from build123d import *

# Parameters (mm, degrees)
PAD_DEPTH       = 10
SKETCH001_W     = 6.633416
SKETCH001_H     = 15.660333
POCKET_DEPTH    = 10.001
SKETCH002_W     = 5.812787
SKETCH002_H     = 16.139036
POCKET001_DEPTH = 2
PAD001_DEPTH    = 10
PAD002_DEPTH    = 10
POCKET002_DEPTH = 5
SKETCH006_W     = 3.933146
SKETCH006_H     = 1.321291
POCKET003_DEPTH = 18.532975


with BuildPart() as part:
    # Sketch → Pad (new body)
    with BuildSketch(Plane.XY):
        Polygon((-15.728714, 20.823448), (11.625568, 20.823448), (23.729843, 16.378376), (23.729843, 12.685549), (12.309424, 6.257293), (12.309424, -2.769621), (17.036469, -7.693392), (17.036469, -16.460198), (-19.695082, -16.460198), (-29.200699, -4.616035), (-29.200699, 13.301021), align=None)
    extrude(amount=PAD_DEPTH)

    # Sketch001 → Pocket (cut, through all)
    with BuildSketch(Plane.XY.offset(10)):
        with Locations((-19.00863, 3.966925)):
            Rectangle(SKETCH001_W, SKETCH001_H)
    extrude(amount=-POCKET_DEPTH, mode=Mode.SUBTRACT)

    # Sketch002 → Pocket001 (cut)
    with BuildSketch(Plane.XY.offset(10)):
        with Locations((-10.392027, 3.590804)):
            Rectangle(SKETCH002_W, SKETCH002_H)
    extrude(amount=-POCKET001_DEPTH, mode=Mode.SUBTRACT)

    # Sketch003 → Pad001 (new body)
    with BuildSketch(Plane.XY.offset(10)):
        Polygon((4.789602, -2.563913), (8.316681, 3.499667), (4.829006, 9.585997), (-2.185748, 9.608747), (-5.712827, 3.545167), (-2.225152, -2.541163), align=None)
    extrude(amount=PAD001_DEPTH)

    # Sketch004 → Pad002 (new body)
    with BuildSketch(Plane.XY.offset(20)):
        with BuildLine():
            ThreePointArc((-1.50189, 5.573991), (-3.143149, 3.932732), (-1.50189, 2.291473))
            Line((-1.50189, 2.291473), (4.379285, 2.291473))
            ThreePointArc((4.379285, 2.291473), (6.020544, 3.932732), (4.379285, 5.573991))
            Line((-1.50189, 5.573991), (4.379285, 5.573991))
        make_face()
    extrude(amount=PAD002_DEPTH)

    # Sketch005 → Pocket002 (cut)
    with BuildSketch(Plane.XZ.offset(16.460198)):
        Polygon((-15.247426, 2.998008), (-12.785538, 7.785009), (-10.05011, 1.972221), align=None)
    extrude(amount=-POCKET002_DEPTH, mode=Mode.SUBTRACT)

    # Sketch006 → Pocket003 (cut, through all)
    with BuildSketch(Plane.XZ.offset(-2.291473)):
        with Locations((1.261401, 26.136292)):
            Rectangle(SKETCH006_W, SKETCH006_H)
    extrude(amount=-POCKET003_DEPTH, mode=Mode.SUBTRACT)


solid = part.part
Read the model definition and answer for the solid it produces. Units are mm, in the model's axes. A direction names the side the tool comes from. Coordinates: 2 decimals unless noted, no trailing zeros. Order: outer loops, then holes, each group sorted by start corner. A loop starts at its lowest first (then second) coordinate and runs counter-clockwise, first axis right, second up. Notation, with made-up numbers: M -4,42 L 48,42 A24 cw 48,65 Z; hole C 40,5.25 d1. An arc over 180 degrees is marked long. Put each result on its own line as item: value. Start each with the question number.
Item 1: Section B-B, the plane x = 1.5 is taken. Determine the outline of the cut face in (y, z).
Item 2: Consider probe 1 along Z at (x, y) = (-7, -3); probe 2 along Y at (x, z) = (4, 15); probe 3 along X at (y, z) = (-14, 7.5). Determine where each line is inside the solid, lowest interval first. Write a range as [from, to].
Item 3: Given pin 1 Ø3 at (x, z) = (-3, 27) entering from -Y; pin 2 Ø1.1 at (y, z) = (4.5, 26) entering from +X; pin 3 Ø1.6 at (y, z) = (7, 9.5) entering from +X; pin 4 Ø3 at (y, z) = (13, 20.5) entering from -X, each flat-ended and moving along its own axis, determine where each tip first touches the part or whether it passes through.
Item 4: Section D-D, the plane z = 7 is taken. Determine the outline of the cut face in (x, y).
Item 5: For faces 1 (the face through (-3.143, 3.969, 24.93)), 2 (the face through (-10, 4, 8)), 3 (the face through (12.309, 2, 5)), determine the directions among +Z, -Z, +X, -X, +Y, -Y from which every point of the face is accessible in a straight line to the end or side of a thin tool.
Item 6: Section C-C, the plane y = -12.5 is taken. Determine the outline of the cut face in (x, z) (3 decimals), plus the area to 3 significant figures.
Item 7: Section A-A, the plane y = 0 is taken. Determine the outline of the cut face in (x, z), plus the area to 3 significant figures.
Item 8: The mould has two halves that part along Y. Classify faces 4 (the face through (1, 5.574, 25)), 5 (the face through (-10, 11.66, 9)), 6 (the face through (-24.4, -10.6, 4.9)): +Y half, -Y half, draft (parallel to the pull), parting line (faces both ways), or undercut.
Computed:
1. outline: M -16.46,0 L 20.82,0 L 20.82,10 L 9.6,10 L 9.6,20 L 5.57,20 L 5.57,25.48 L 2.29,25.48 L 2.29,20 L -2.55,20 L -2.55,10 L -16.46,10 Z; M 2.29,26.8 L 5.57,26.8 L 5.57,30 L 2.29,30 Z
2. probe 1: z = [0, 10]
2. probe 2: y = [-2.56, 9.59]
2. probe 3: x = [-21.67, -12.93], [-12.65, 17.04]
3. pin 1: stops at y = 2.29
3. pin 2: stops at x = 6.02
3. pin 3: stops at x = 15.05
3. pin 4: passes through
4. outline: M -29.2,-4.62 L -19.7,-16.46 L -13.19,-16.46 L -13.19,-11.46 L -12.42,-11.46 L -12.42,-16.46 L 17.04,-16.46 L 17.04,-7.69 L 12.31,-2.77 L 12.31,6.26 L 23.73,12.69 L 23.73,16.38 L 11.63,20.82 L -15.73,20.82 L -29.2,13.3 Z; hole M -22.33,-3.86 L -15.69,-3.86 L -15.69,11.8 L -22.33,11.8 Z
5. face 1: +Z, -X
5. face 2: +Z
5. face 3: +Z, -Z, +X
6. outline: M -22.873,0 L 17.036,0 L 17.036,10 L -22.873,10 Z; hole M -15.247,2.998 L -10.05,1.972 L -12.786,7.785 Z
6. area: 385 mm2
7. outline: M -29.2,0 L -22.33,0 L -22.33,10 L -29.2,10 Z; M -15.69,0 L 12.31,0 L 12.31,10 L 6.28,10 L 6.28,20 L -3.68,20 L -3.68,10 L -7.49,10 L -7.49,8 L -13.3,8 L -13.3,10 L -15.69,10 Z
7. area: 437 mm2
8. face 4: +Y half
8. face 5: undercut
8. face 6: -Y half
